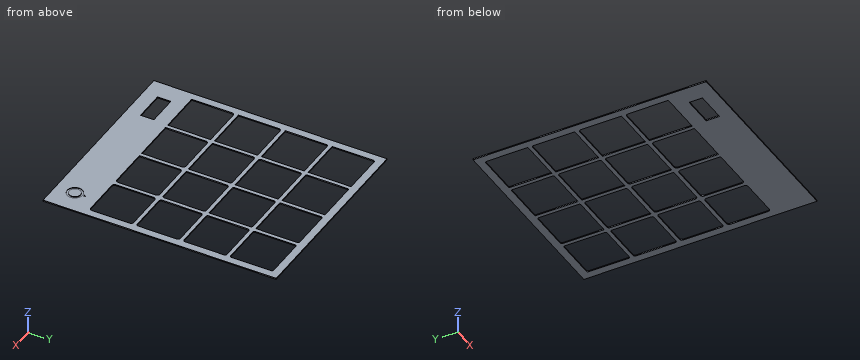
```python
from build123d import *

# Parameters (mm, degrees)
SKETCH_W                     = 520
SKETCH_H                     = 610
PAD_DEPTH                    = 3
SKETCH001_W                  = 112.5
SKETCH001_H                  = 112.5
POCKET_DEPTH                 = 5
SKETCH001_LINEARPATTERN_2_W  = 112.5
SKETCH001_LINEARPATTERN_2_H  = 112.5
POCKET_LINEARPATTERN_2_DEPTH = 5
SKETCH001_LINEARPATTERN_3_W  = 112.5
SKETCH001_LINEARPATTERN_3_H  = 112.5
POCKET_LINEARPATTERN_3_DEPTH = 5
SKETCH001_LINEARPATTERN_4_W  = 112.5
SKETCH001_LINEARPATTERN_4_H  = 112.5
POCKET_LINEARPATTERN_4_DEPTH = 5
LINEARPATTERN001_COUNT       = 4
LINEARPATTERN001_PITCH       = 122.5
FILLET_R                     = 4
FILLET001_R                  = 5
FILLET002_R                  = 6
FILLET003_R                  = 7
SKETCH002_R                  = 20
SKETCH002_R_2                = 15
POCKET001_DEPTH              = 1
SKETCH003_W                  = 80
SKETCH003_H                  = 35
POCKET002_DEPTH              = 5


with BuildPart() as part:
    # Sketch → Pad (new body)
    with BuildSketch(Plane.XY):
        with Locations((0, -45)):
            Rectangle(SKETCH_W, SKETCH_H)
    extrude(amount=-PAD_DEPTH)

    # Sketch001 (on Face5 of Pad) → Pocket (cut)
    with BuildSketch(Plane.XY):
        with Locations((-183.75, 183.75)):
            Rectangle(SKETCH001_W, SKETCH001_H)
    pocket = extrude(amount=-POCKET_DEPTH, mode=Mode.SUBTRACT)

    # Sketch001 LinearPattern 2 → Pocket LinearPattern 2 (cut)
    with BuildSketch(Plane(origin=(122.5, 0, 0), x_dir=(1, 0, 0), z_dir=(0, 0, 1))):
        with Locations((-183.75, 183.75)):
            Rectangle(SKETCH001_LINEARPATTERN_2_W, SKETCH001_LINEARPATTERN_2_H)
    pocket_linearpattern_2 = extrude(amount=-POCKET_LINEARPATTERN_2_DEPTH, mode=Mode.SUBTRACT)

    # Sketch001 LinearPattern 3 → Pocket LinearPattern 3 (cut)
    with BuildSketch(Plane(origin=(245, 0, 0), x_dir=(1, 0, 0), z_dir=(0, 0, 1))):
        with Locations((-183.75, 183.75)):
            Rectangle(SKETCH001_LINEARPATTERN_3_W, SKETCH001_LINEARPATTERN_3_H)
    pocket_linearpattern_3 = extrude(amount=-POCKET_LINEARPATTERN_3_DEPTH, mode=Mode.SUBTRACT)

    # Sketch001 LinearPattern 4 → Pocket LinearPattern 4 (cut)
    with BuildSketch(Plane(origin=(367.5, 0, 0), x_dir=(1, 0, 0), z_dir=(0, 0, 1))):
        with Locations((-183.75, 183.75)):
            Rectangle(SKETCH001_LINEARPATTERN_4_W, SKETCH001_LINEARPATTERN_4_H)
    pocket_linearpattern_4 = extrude(amount=-POCKET_LINEARPATTERN_4_DEPTH, mode=Mode.SUBTRACT)

    # LinearPattern001: Pocket, Pocket LinearPattern 2, Pocket LinearPattern 3, Pocket LinearPattern 4 ×4
    with Locations(*[(0, -i * LINEARPATTERN001_PITCH, 0) for i in range(1, LINEARPATTERN001_COUNT)]):
        add(pocket, mode=Mode.SUBTRACT)
        add(pocket_linearpattern_2, mode=Mode.SUBTRACT)
        add(pocket_linearpattern_3, mode=Mode.SUBTRACT)
        add(pocket_linearpattern_4, mode=Mode.SUBTRACT)

    # Fillet
    fillet_edges = [part.edges().sort_by_distance(p)[0] for p in [
        (-240, 240, -1.5),
        (-117.5, 240, -1.5),
        (-117.5, 127.5, -1.5),
        (5, 240, -1.5),
        (117.5, 240, -1.5),
        (5, 127.5, -1.5),
        (127.5, 127.5, -1.5),
        (127.5, 240, -1.5),
        (240, 240, -1.5),
        (240, 127.5, -1.5),
    ]]
    fillet(fillet_edges, radius=FILLET_R)

    # Fillet001
    fillet001_edges = [part.edges().sort_by_distance(p)[0] for p in [
        (-240, 117.5, -1.5),
        (-117.5, 117.5, -1.5),
        (5, 117.5, -1.5),
        (127.5, 117.5, -1.5),
        (240, 117.5, -1.5),
        (240, 5, -1.5),
        (127.5, 5, -1.5),
        (117.5, 117.5, -1.5),
        (5, 5, -1.5),
        (-117.5, 5, -1.5),
    ]]
    fillet(fillet001_edges, radius=FILLET001_R)

    # Fillet002
    fillet002_edges = [part.edges().sort_by_distance(p)[0] for p in [
        (-240, -5, -1.5),
        (-117.5, -5, -1.5),
        (5, -5, -1.5),
        (127.5, -5, -1.5),
        (240, -5, -1.5),
        (240, -117.5, -1.5),
        (127.5, -117.5, -1.5),
        (117.5, -5, -1.5),
        (117.5, -117.5, -1.5),
        (-5, -5, -1.5),
    ]]
    fillet(fillet002_edges, radius=FILLET002_R)

    # Fillet003
    fillet003_edges = [part.edges().sort_by_distance(p)[0] for p in [
        (-240, -127.5, -1.5),
        (-117.5, -127.5, -1.5),
        (5, -127.5, -1.5),
        (127.5, -127.5, -1.5),
        (240, -127.5, -1.5),
        (240, -240, -1.5),
        (127.5, -240, -1.5),
        (117.5, -127.5, -1.5),
        (117.5, -240, -1.5),
        (-5, -127.5, -1.5),
    ]]
    fillet(fillet003_edges, radius=FILLET003_R)

    # Sketch002 (on Face1 of Fillet003) → Pocket001 (cut)
    with BuildSketch(Plane.XY):
        with Locations((200, -300)):
            Circle(SKETCH002_R)
        with Locations((200, -300)):
            Circle(SKETCH002_R_2, mode=Mode.SUBTRACT)
        Polygon((200.37776, -271.535898), (197.37776, -276.732051), (203.37776, -276.732051), align=None)
    extrude(amount=-POCKET001_DEPTH, mode=Mode.SUBTRACT)

    # Sketch003 (on Face1 of Pocket001) → Pocket002 (cut)
    with BuildSketch(Plane.XY):
        with Locations((-170, -295)):
            Rectangle(SKETCH003_W, SKETCH003_H)
    extrude(amount=-POCKET002_DEPTH, mode=Mode.SUBTRACT)


solid = part.part
```
The listing builds one solid part. Answer for the finished solid, in the listing's coordinates (mm). Coordinates: 2 decimals unless noted, no trailing zeros. Loops run counter-clockwise (first coordinate to the right, second up) from the corner with the lowest first, then second, coordinate; pieces in that order, holes last. Notation, with made-up numbers: (-33, 67.25) - (-27, 67.25) arc R31 cw to (-27, 94.25) - close; hole circle Ø11 at (52.5, -32.75). An arc over 180 degrees is marked (long way). Use a Markdown table: item, result. Add a question column.
1) Find the intervals of material crossed by line 1 (X direction, y = -101.5, z = -1.6); line 2 (Y direction, x = 57.5, z = -1.55); line 3 (Y direction, x = -199.5, z = -1.15), in increasing order.
2) The part is cut by section D-D, the plane x = -160.5. Give the vertices of the cut face in (y, z).
3) The part is cut by section C-C, the plane y = 83.5. Give the vertices of the cut face in (x, z), and give its area (3 significant figures).
4) Given pin 1 (6 mm diameter, centred on x = 131, y = -274, fed in from +Z), flat-ended and moving along its own axis, determine where the tip first touches the part or whether it passes through.
5) The part is cut by section A-A, the plane x = 170. Give the vertices of the cut face in (y, z), and give its area (3 significant figures).
6) The part is cut by section B-B, the plane y = -300. Give the vertices of the cut face in (x, z).
Here are the results:
| question | item | result |
|---|---|---|
| 1 | line 1 | x = -260 to -240, -127.5 to -117.5, -5 to 5, 117.5 to 127.5, 240 to 260 |
| 1 | line 2 | y = -350 to -240, -127.5 to -117.5, -5 to 5, 117.5 to 127.5, 240 to 260 |
| 1 | line 3 | y = -350 to -312.5, -277.5 to -240, -127.5 to -117.5, -5 to 5, 117.5 to 127.5, 240 to 260 |
| 2 | outline | (-350, -3) - (-312.5, -3) - (-312.5, 0) - (-350, 0) - close; (-277.5, -3) - (-240, -3) - (-240, 0) - (-277.5, 0) - close; (-127.5, -3) - (-117.5, -3) - (-117.5, 0) - (-127.5, 0) - close; (-5, -3) - (5, -3) - (5, 0) - (-5, 0) - close; (117.5, -3) - (127.5, -3) - (127.5, 0) - (117.5, 0) - close; (240, -3) - (260, -3) - (260, 0) - (240, 0) - close |
| 3 | outline | (-260, -3) - (-240, -3) - (-240, 0) - (-260, 0) - close; (-127.5, -3) - (-117.5, -3) - (-117.5, 0) - (-127.5, 0) - close; (-5, -3) - (5, -3) - (5, 0) - (-5, 0) - close; (117.5, -3) - (127.5, -3) - (127.5, 0) - (117.5, 0) - close; (240, -3) - (260, -3) - (260, 0) - (240, 0) - close |
| 3 | area | 210 mm^2 |
| 4 | pin 1 | stops at z = 0 |
| 5 | outline | (-350, -3) - (-240, -3) - (-240, 0) - (-350, 0) - close; (-127.5, -3) - (-117.5, -3) - (-117.5, 0) - (-127.5, 0) - close; (-5, -3) - (5, -3) - (5, 0) - (-5, 0) - close; (117.5, -3) - (127.5, -3) - (127.5, 0) - (117.5, 0) - close; (240, -3) - (260, -3) - (260, 0) - (240, 0) - close |
| 5 | area | 480 mm^2 |
| 6 | outline | (-260, -3) - (-210, -3) - (-210, 0) - (-260, 0) - close; (-130, -3) - (260, -3) - (260, 0) - (220, 0) - (220, -1) - (215, -1) - (215, 0) - (185, 0) - (185, -1) - (180, -1) - (180, 0) - (-130, 0) - close |
